Geometry: final body of the model. Coordinates: model frame, mm. Face numbers are marked on the shaded views. A direction names the side the tool comes from. Coordinates: 2 decimals unless noted, no trailing zeros. Order: outer loops, then holes, each group sorted by start corner. A loop starts at its lowest first (then second) coordinate and runs counter-clockwise, first axis right, second up. Notation, with made-up numbers: M 1,53.5 L 33,53.5 A22 cw 33,60.5 Z; hole C 12.25,-4.75 d5. An arc over 180 degrees is marked long. Write item = value, one per line.
from build123d import *

# Parameters (mm, degrees)
F0_W     = 119.3591766059
F0_H     = 25.3895912319
F1_DEPTH = 73.66
F3_DEPTH = 119.38
F5_DEPTH = 35.814
F6_DEPTH = 17.78


with BuildPart() as f1:
    # F0 (on Front) → F1 (new body)
    with BuildSketch(Plane.XZ):
        with Locations((-5.246559158, 12.694795616)):
            Rectangle(F0_W, F0_H)
    extrude(amount=F1_DEPTH)

    # F2 (on face) → F3 (join)
    with BuildSketch(Plane.YZ.offset(54.433029145)):
        Polygon((-38.0689874291, 25.3895912319), (0, 25.3895912319), (-38.0689874291, 45.67636922), align=None)
        Polygon((-76.133325696, 25.3895912319), (-38.0689874291, 25.3895912319), (-38.0689874291, 45.67636922), align=None)
    extrude(amount=-F3_DEPTH)

    # F4 (on face) → F5 (join)
    with BuildSketch(Plane.XZ.offset(73.66)):
        Polygon((-34.4408005476, 25.3895912319), (-21.6549783945, 25.3895912319), (-34.4408005476, 33.0080874264), align=None)
        Polygon((27.8254915029, 25.3895912319), (54.433029145, 25.3895912319), (27.8254915029, 45.8136871457), align=None)
        Polygon((1.1622435413, 25.3895912319), (27.8254915029, 25.3895912319), (27.8254915029, 45.8136871457), align=None)
        Polygon((-47.1603758633, 25.3895912319), (-34.4408005476, 25.3895912319), (-34.4408005476, 33.0080874264), align=None)
    extrude(amount=-F5_DEPTH)

    # F4 (on face) → F6 (join)
    with BuildSketch(Plane.XZ.offset(73.66)):
        Polygon((54.433029145, 0), (54.433029145, 25.3895912319), (27.8254915029, 25.3895912319), (1.1622435413, 25.3895912319), (0, 0), align=None)
        Polygon((27.8254915029, 25.3895912319), (54.433029145, 25.3895912319), (27.8254915029, 45.8136871457), align=None)
        Polygon((1.1622435413, 25.3895912319), (27.8254915029, 25.3895912319), (27.8254915029, 45.8136871457), align=None)
        Polygon((-34.4408005476, 33.0080874264), (-47.1603758633, 25.3895912319), (-34.4408005476, 25.3895912319), align=None)
        Polygon((-34.4408005476, 25.3895912319), (-47.1603758633, 25.3895912319), (-47.1603758633, 0), (-21.6549783945, 0), (-21.6549783945, 25.3895912319), align=None)
        Polygon((-34.4408005476, 33.0080874264), (-34.4408005476, 25.3895912319), (-21.6549783945, 25.3895912319), align=None)
    extrude(amount=F6_DEPTH)


solid = f1.part
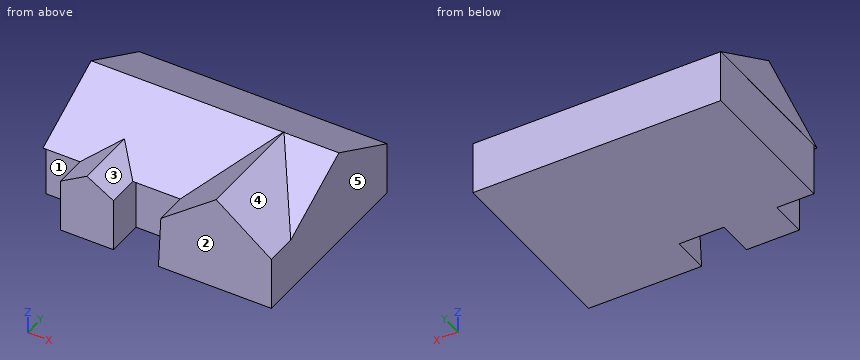
1) Section C-C, the plane z = 41. Return loops of the section in (x, y), and give its area (3 significant figures).
Numbers:
outline = M -64.95,-46.84 L 21.54,-46.84 L 21.54,-91.44 L 34.1,-91.44 L 34.1,-46.84 L 54.43,-46.84 L 54.43,-29.29 L -64.95,-29.29 Z
area = 2,660 mm²
2) Line query: L1, parallel to X at y = -31, z = 11; L2, parallel to X at y = -77.5, z = 17.5; L3, parallel to Y at x = -21.5, z = 19. Output: solid intervals per line, ascending.
Numbers:
L1 = -64.93 to 54.43
L2 = -47.16 to -21.65, 0.8 to 54.43
L3 = -73.66 to 0
3) Section A-A, the plane y = -78. Return loops of the section in (x, z).
Numbers:
outline = M -47.16,0 L -21.65,0 L -21.65,25.39 L -34.44,33.01 L -47.16,25.39 Z; M 0,0 L 54.43,0 L 54.43,25.39 L 27.83,45.81 L 1.16,25.39 Z
4) Section B-B, the plane x = -5. Return loops of the section in (y, z), and give its area (3 significant figures).
Numbers:
outline = M -76.13,25.39 L -73.66,25.39 L -73.66,0 L 0,0 L 0,25.39 L -38.07,45.68 Z
area = 2,640 mm²
5) Pin query (flat end, axial travel): pin 1 (5 mm diameter, centred on x = -46.5, y = -20.5, fed in from +Z); pin 2 (5.5 mm diameter, centred on y = -79.5, z = 11.5, fed in from -X); pin 3 (5.5 mm diameter, centred on x = -57.5, z = 8.5, fed in from -Y). Return the tip coordinate at first contact, or that it passes through.
Numbers:
pin_1 = 37.65
pin_2 = -47.16
pin_3 = -73.66
6) Set-up query: the marked faces 1, 2, 3, 4 and 5. Return all of +Z, -Z, +X, -X, +Y, -Y with unobstructed straight access to the full face (end or side cutting, diameter ignored); none if empty.
Numbers:
face_1 = -Z, -X, -Y
face_2 = +Z, -Z, +X, -X, -Y
face_3 = +Z, -Y
face_4 = +Z, +X, -Y
face_5 = +Z, -Z, +X, +Y, -Y
